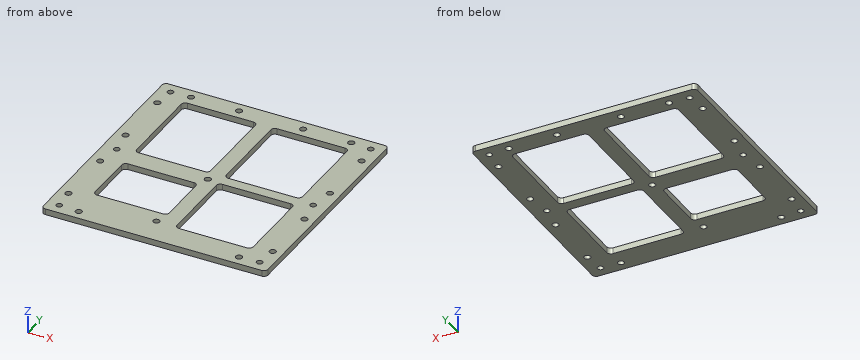
Autodesk Inventor part; units mm, degrees
ref_plane "YZ Plane" through (0, 0, 0) normal (1, 0, 0) x (0, 1, 0)
ref_plane "XZ Plane" through (0, 0, 0) normal (0, 1, 0) x (-1, 0, 0)
ref_plane "XY Plane" through (0, 0, 0) normal (0, 0, 1) x (1, 0, 0)
sketch "Sketch1" plane through (0, 0, 0) normal (0, 0, 1) x (1, 0, 0)
  line L0 (-56, -58) -> (56, -58)
  line L1 (56, -58) -> (56, 58)
  line L2 (56, 58) -> (-56, 58)
  line L3 (-56, 58) -> (-56, -58)
  line L4 (-56, -58) -> (56, 58) construction
  line L5 (56, -58) -> (-56, 58) construction
  point P0 (0, 0)
  dimension "d0" = 116
  dimension "d1" = 112
extrude "Extrusion1" add sketch "Sketch1" along normal blind 3
sketch "Sketch2" plane through (0, 0, 3) normal (0, 0, 1) x (1, 0, 0)
  line L0 (-78.4, 0) -> (78.4, 0) construction
  line L1 (0, 81.2) -> (0, -81.2) construction
  circle A0 centre (-50, 52.5) radius 1.5
  circle A1 centre (50, 52.5) radius 1.5
  circle A2 centre (-50, -52.5) radius 1.5
  circle A3 centre (50, -52.5) radius 1.5
  circle A4 centre (49, 0) radius 1.5
  line L2 (78.4, 0) -> (-78.4, 0) construction
  circle A5 centre (-49, 0) radius 1.5
  point P0 (0, 0)
  dimension "d4" = 3
  dimension "d5" = 100
  dimension "d6" = 105
  dimension "d44" = 3
  dimension "d45" = 98
extrude "Extrusion2" cut sketch "Sketch2" against normal through all
fillet "Fillet1" radius 2 4 edges at (-56, 58, 1.5) (-56, -58, 1.5) (56, -58, 1.5) (56, 58, 1.5)
sketch "Sketch3" plane through (0, 0, 3) normal (0, 0, 1) x (1, 0, 0)
  line L0 (22.6276, -51.0248) -> (22.6276, 2.6708)
  line L1 (47.313, -24.177) -> (-2.0522, -24.177)
  line L2 (-47.3418, -22.8308) -> (2.0866, -22.8308)
  line L3 (-22.6276, -42.0332) -> (-22.6276, -3.6284)
  line L4 (2.0578, 24.9075) -> (-47.3074, 24.9075)
  line L5 (-22.6276, -5.5598) -> (-22.6276, 54.3588)
  line L6 (47.313, 24.9075) -> (-2.0522, 24.9075)
  line L7 (22.6276, -5.5598) -> (22.6276, 54.3588)
  line L8 (41.6304, -3.677) -> (3.6304, -3.677)
  line L9 (3.6304, -3.677) -> (3.6304, -44.677)
  line L10 (3.6304, -44.677) -> (41.6304, -44.677)
  line L11 (41.6304, -44.677) -> (41.6304, -3.677)
  line L12 (41.6304, -3.677) -> (3.6304, -44.677) construction
  line L13 (3.6304, -3.677) -> (41.6304, -44.677) construction
  line L14 (-4.1276, -8.3308) -> (-41.1276, -8.3308)
  line L15 (-41.1276, -8.3308) -> (-41.1276, -37.3308)
  line L16 (-41.1276, -37.3308) -> (-4.1276, -37.3308)
  line L17 (-4.1276, -37.3308) -> (-4.1276, -8.3308)
  line L18 (-4.1276, -8.3308) -> (-41.1276, -37.3308) construction
  line L19 (-41.1276, -8.3308) -> (-4.1276, -37.3308) construction
  line L20 (-4.1276, 47.9075) -> (-41.1276, 47.9075)
  line L21 (-41.1276, 47.9075) -> (-41.1276, 1.9075)
  line L22 (-41.1276, 1.9075) -> (-4.1276, 1.9075)
  line L23 (-4.1276, 1.9075) -> (-4.1276, 47.9075)
  line L24 (-4.1276, 47.9075) -> (-41.1276, 1.9075) construction
  line L25 (-41.1276, 47.9075) -> (-4.1276, 1.9075) construction
  line L26 (41.6248, 47.9075) -> (3.6304, 47.9075)
  line L27 (3.6304, 47.9075) -> (3.6304, 1.9075)
  line L28 (3.6304, 1.9075) -> (41.6248, 1.9075)
  line L29 (41.6248, 1.9075) -> (41.6248, 47.9075)
  line L30 (41.6248, 47.9075) -> (3.6304, 1.9075) construction
  line L31 (3.6304, 47.9075) -> (41.6248, 1.9075) construction
  point P0 (0, 0)
  point P1 (22.6304, -24.177)
  point P2 (-22.6276, -22.8308)
  point P3 (-22.6276, 24.9075)
  point P4 (22.6276, 24.9075)
  point P5 (-4.1276, -22.8308)
  point P6 (-22.6276, -22.8308)
  point P7 (-22.6276, -8.3308)
  dimension "d10" = 41
  dimension "d11" = 38
  dimension "d12" = 46
  dimension "d13" = 29
  dimension "d14" = 37
  dimension "d15" = 37
extrude "Extrusion3" cut sketch "Sketch3" against normal through all
fillet "Fillet2" radius 2 16 edges at (41.6304, -44.677, 1.5) (3.6304, -44.677, 1.5) (-4.1276, -37.3308, 1.5) (-41.1276, -37.3308, 1.5) (-41.1276, -8.3308, 1.5) (-41.1276, 1.9075, 1.5) (-41.1276, 47.9075, 1.5) (-4.1276, 47.9075, 1.5) (41.6248, 47.9075, 1.5) (3.6304, 47.9075, 1.5) (-4.1276, 1.9075, 1.5) (3.6304, 1.9075, 1.5) (41.6248, 1.9075, 1.5) (41.6304, -3.677, 1.5) (3.6304, -3.677, 1.5) (-4.1276, -8.3308, 1.5)
sketch "Sketch5" plane through (0, 0, 3) normal (0, 0, 1) x (1, 0, 0)
  circle A0 centre (-2, -3) radius 1.6
  circle A1 centre (-6, -44) radius 1.6
  circle A2 centre (40, -53) radius 1.6
  circle A3 centre (51, -42) radius 1.6
  circle A4 centre (51, -12) radius 1.6
  line L0 (56, -56) -> (56, 56) construction
  line L1 (-54, -58) -> (54, -58) construction
  line L2 (0, 81.2) -> (0, -81.2) construction
  line L3 (-78.4, 0) -> (78.4, 0) construction
  circle A5 centre (-40, -53) radius 1.6
  circle A6 centre (-51, -42) radius 1.6
  circle A7 centre (-51, -12) radius 1.6
  circle A8 centre (40, 53) radius 1.6
  circle A9 centre (51, 42) radius 1.6
  circle A10 centre (51, 12) radius 1.6
  line L4 (-54, 58) -> (54, 58) construction
  circle A11 centre (-51, 12) radius 1.6
  circle A12 centre (-51, 42) radius 1.6
  circle A13 centre (-40, 53) radius 1.6
  circle A14 centre (16, 53) radius 1.6
  circle A15 centre (-16, 53) radius 1.6
  point P0 (0, 0)
  point P1 (-56, -56)
  point P2 (-56, 56)
  dimension "d19" = 44
  dimension "d20" = 6
  dimension "d21" = 3
  dimension "d22" = 2
  dimension "d23" = 5
  dimension "d24" = 5
  dimension "d25" = 5
  dimension "d27" = 3.2
  dimension "d28" = 3.2
  dimension "d29" = 3.2
  dimension "d31" = 3.2
  dimension "d32" = 3.2
  dimension "d33" = 16
  dimension "d34" = 16
  dimension "d35" = 12
  dimension "d36" = 3.2
  dimension "d37" = 3.2
  dimension "d38" = 5
  dimension "d39" = 5
  dimension "d40" = 16
  dimension "d41" = 16
extrude "Extrusion4" cut sketch "Sketch5" against normal through all
equation "\"d44\" = d4"
equation "\"d24\" = d23"
equation "\"d25\" = d23"
equation "\"d28\" = d27"
equation "\"d29\" = d27"
equation "\"d31\" = d27"
equation "\"d32\" = d27"
equation "\"d36\" = d27"
equation "\"d37\" = d27"
equation "\"d38\" = d23"
equation "\"d39\" = d23"
equation "\"d40\" = d34"
equation "\"d41\" = d34"
properties part number "AssemblyPlate"
Read the model definition and answer for the solid it produces. Units are mm, in the model's axes. Coordinates: 2 decimals unless noted, no trailing zeros. Loops run counter-clockwise (first coordinate to the right, second up) from the corner with the lowest first, then second, coordinate; pieces in that order, holes last. Notation, with made-up numbers: (82.25, 27.25) - (139.25, 27.25) arc R19 ccw to (139.25, 62.25) - close; hole circle Ø2 at (-4.5, -25). An arc over 180 degrees is marked (long way). Answer in a Markdown table with one row per item.
Q1. Find section D-D on z = 1.1. Count the separate pieces of the cut face and the enclosed holes in it, plus the area to 3 significant figures.
Here are the results:
| item | result |
|---|---|
| separate pieces | 1 |
| enclosed holes | 26 |
| area | 6,750 mm^2 |
Q2. Find section B-B on x = 16. Write down the section's boundary in (y, z), plus the area to 3 significant figures.
Here are the results:
| item | result |
|---|---|
| outline | (-58, 0) - (-44.68, 0) - (-44.68, 3) - (-58, 3) - close; (-3.68, 0) - (1.91, 0) - (1.91, 3) - (-3.68, 3) - close; (47.91, 0) - (51.4, 0) - (51.4, 3) - (47.91, 3) - close; (54.6, 0) - (58, 0) - (58, 3) - (54.6, 3) - close |
| area | 77.4 mm^2 |
Q3. Straight lines are drawn through the part: line 1 along Y through (x, z) = (-24, 1.15); line 2 along X through (y, z) = (35.5, 2); line 3 along Y through (x, z) = (-2, 1). For each, find the intervals that lie inside material, in ascending order. Write a range as [from, to].
Here are the results:
| item | result |
|---|---|
| line 1 | y = [-58, -37.33], [-8.33, 1.91], [47.91, 58] |
| line 2 | x = [-56, -41.13], [-4.13, 3.63], [41.62, 56] |
| line 3 | y = [-58, -4.6], [-1.4, 58] |
Q4. Find section C-C on x = -27. Write down the section's boundary in (y, z).
Here are the results:
| item | result |
|---|---|
| outline | (-58, 0) - (-37.33, 0) - (-37.33, 3) - (-58, 3) - close; (-8.33, 0) - (1.91, 0) - (1.91, 3) - (-8.33, 3) - close; (47.91, 0) - (58, 0) - (58, 3) - (47.91, 3) - close |
Q5. Find section A-A on x = 33.5. Write down the section's boundary in (y, z).
Here are the results:
| item | result |
|---|---|
| outline | (-58, 0) - (-44.68, 0) - (-44.68, 3) - (-58, 3) - close; (-3.68, 0) - (1.91, 0) - (1.91, 3) - (-3.68, 3) - close; (47.91, 0) - (58, 0) - (58, 3) - (47.91, 3) - close |
Q6. Given P1, Ø2.5, axis at x = 40, y = -53, coming from the +Z side, flat-ended and moving along its own axis, determine where the tip first touches the part or whether it passes through.
Here are the results:
| item | result |
|---|---|
| P1 | passes through |
